Source: CAD feature listing. Evaluate the final solid. Frame: model axes, mm. Face numbers are marked on the shaded views. Round coordinates to 2 decimals unless told otherwise and drop trailing zeros. Order: outer loops, then holes, each group sorted by start corner. A loop starts at its lowest first (then second) coordinate and runs counter-clockwise, first axis right, second up. Notation, with made-up numbers: (55.25, 37) -> (85.25, 37) arc R30 ccw to (85.25, 73) -> close; hole circle Ø1 at (20.5, 10.25). An arc over 180 degrees is marked (long way). Answer as CSV lines item,"result". Start each with the question number.
(1) Section query D-D (z = 22.25). Output: boundary loops of the cut face in (x, y) (3 decimals), plus the area to 3 significant figures.
(2) Contact query for flat-ended pins moving along their axis: P1, Ø1, axis at y = -6, z = 13, coming from the -X side; P2, Ø6, axis at x = 3, z = 21.5, coming from the +Y side; P3, Ø2, axis at x = 2.5, z = 14, coming from the -Y side. Output: stop coordinate, or through.
(3) Section query C-C (z = 14). Output: boundary loops of the cut face in (x, y) (3 decimals).
(4) Section query A-A (y = 0). Output: boundary loops of the cut face in (x, z) (3 decimals), plus the area to 3 significant figures.
(5) Pull-direction query (X, two-part tool) for the marked faces 1 and 2; classes: +X half, -X half, draft (parallel to the pull), parting line (faces both ways), or undercut.
(6) Line query: line 1 along Y through (x, z) = (0, 19) (3 decimals); line 2 along X through (y, z) = (0.5, 3); line 3 along X through (y, z) = (-4.5, 12.25). Output: solid intervals per line, ascending. Write a range as from..to.
```python
from build123d import *

# Parameters (mm, degrees)
F0_R     = 15.875
F0_R_2   = 13.335
F1_DEPTH = 25.4
F2_SIZE2 = 1.5748
F2_SIZE  = 6.35
F3_R     = 0.508


with BuildPart() as f1:
    # F0 (on Top) → F1 (new body)
    with BuildSketch(Plane.XY):
        Circle(F0_R)
        Circle(F0_R_2, mode=Mode.SUBTRACT)
    extrude(amount=F1_DEPTH)

    # F2
    f2_edges = [f1.edges().sort_by_distance(p)[0] for p in [
        (-15.875, 0, 25.4),
    ]]
    f2_side = f1.faces().sort_by_distance((-15.875, 0, 12.7))[0]
    chamfer(f2_edges, length=F2_SIZE, length2=F2_SIZE2, reference=f2_side)

    # F3
    f3_edges = [f1.edges().sort_by_distance(p)[0] for p in [
        (-14.3002, 0, 25.4),
        (-13.335, 0, 25.4),
        (-15.875, 0, 0),
        (-13.335, 0, 0),
    ]]
    fillet(f3_edges, radius=F3_R)


solid = f1.part
```
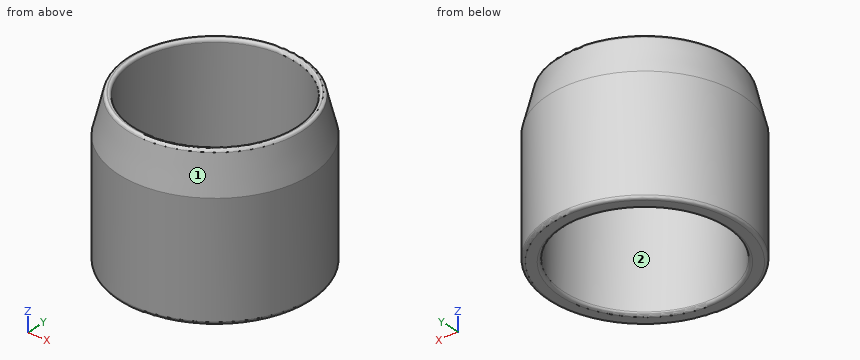
Answer block:
1,outline,"circle Ø30.163 at (0, 0); hole circle Ø26.67 at (0, 0)"
1,area,"156 mm2"
2,P1,"x = -14.89"
2,P2,"y = 15.82"
2,P3,"y = -15.8"
3,outline,"circle Ø31.75 at (0, 0); hole circle Ø26.67 at (0, 0)"
4,outline,"(-15.875, 0.508) arc R0.508 ccw to (-15.367, 0) -> (-13.843, 0) arc R0.508 ccw to (-13.335, 0.508) -> (-13.335, 24.892) arc R0.508 ccw to (-13.843, 25.4) -> (-13.903, 25.4) arc R0.508 ccw to (-14.396, 25.014) -> (-15.875, 19.05) -> close; (13.335, 0.508) arc R0.508 ccw to (13.843, 0) -> (15.367, 0) arc R0.508 ccw to (15.875, 0.508) -> (15.875, 19.05) -> (14.396, 25.014) arc R0.508 ccw to (13.903, 25.4) -> (13.843, 25.4) arc R0.508 ccw to (13.335, 24.892) -> close"
4,area,"119 mm2"
5,face 1,"parting line"
5,face 2,"undercut"
6,line 1,"-15.875..-13.335, 13.335..15.875"
6,line 2,"-15.87..-13.33, 13.33..15.87"
6,line 3,"-15.22..-12.55, 12.55..15.22"
